The model under review builds one solid part; all positions refer to its coordinate system, in mm. Face numbers are marked on the shaded views. A direction names the side the tool comes from. Round coordinates to 2 decimals unless told otherwise and drop trailing zeros. Order: outer loops, then holes, each group sorted by start corner. A loop starts at its lowest first (then second) coordinate and runs counter-clockwise, first axis right, second up.
1) To check wall thickness, follow L1, parallel to Y at x = -13.8, z = 6.25; L2, parallel to Y at x = 9, z = -1.25; L3, parallel to Z at x = 6, y = 9.5. State the ranges of each line that lie inside material, in increasing order.
2) Consider section D-D (x = -8). Give the boundary of the cut face in (y, z).
3) Consider section A-A (x = -13.8). Give the boundary of the cut face in (y, z).
4) Consider section C-C (z = 3.75). Give the boundary of the cut face in (x, y).
5) Clearance check with flat-ended pins moving along their axes: P1, Ø5, axis at y = 12.5, z = 5.5, coming from the -X side; P2, Ø1, axis at y = 11.5, z = 6.5, coming from the +X side; P3, Ø1.8, axis at x = 13.8, y = 25.4, coming from the +Z side; P4, Ø3, axis at x = -10, z = 12, coming from the +Y side. State where each tip first meets the part, or that it passes through.
6) Consider section B-B (y = 25.4). Give the boundary of the cut face in (x, z), then the cut area to 3 significant figures.
7) Mouldability with a two-part tool opening along X and no side actions: class the marked faces 4, 5, 6 and 7 as pulls with the +X half, pulls with the -X half, needs draft (parallel to the pull), parting line crosses it, or undercut.
8) Machinability: for the marked faces 1, 2 and 3, which of the approach directions +Z, -Z, +X, -X, +Y, -Y give a long, thin tool a straight path to every point of the face, cutting with its end or side? Answer none if there is none.
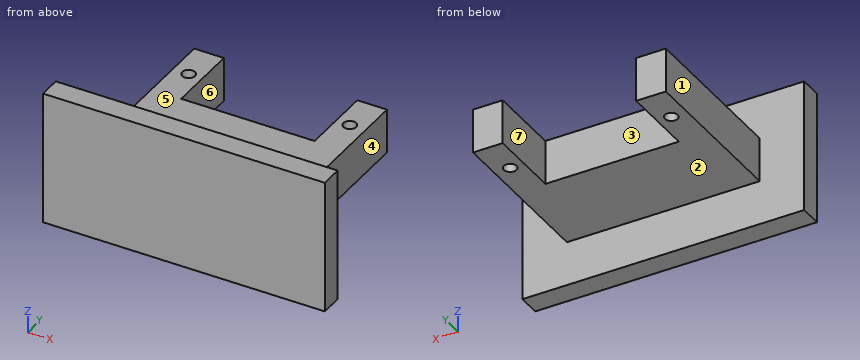
from build123d import *

# Parameters (mm, degrees)
BOSS_EXTRUDE4_DEPTH  = 7.62
SKETCH7_W            = 48.26
SKETCH7_H            = 22.86
BOSS_EXTRUDE5_DEPTH  = 3.81
M2_CLEARANCE_HOLE1_D = 2.2


with BuildPart() as part:
    # Sketch6 → Boss-Extrude4 (new body)
    with BuildSketch(Plane.XY):
        Polygon((-11.43, 19.05), (11.43, 19.05), (11.43, 31.75), (16.51, 31.75), (16.51, 0), (-16.51, 0), (-16.51, 31.75), (-11.43, 31.75), align=None)
    extrude(amount=BOSS_EXTRUDE4_DEPTH)

    # Sketch7 → Boss-Extrude5 (add)
    with BuildSketch(Plane(origin=(0, 0, 0), x_dir=(1, 0, 0), z_dir=(0, 1, 0))):
        with Locations((0, -3.81)):
            Rectangle(SKETCH7_W, SKETCH7_H)
    extrude(amount=BOSS_EXTRUDE5_DEPTH)

    # M2 Clearance Hole1 (through all)
    with Locations(Plane(origin=(0, 0, 0), x_dir=(-1, 0, 0), z_dir=(0, 0, -1))):
        with Locations((-13.8, 25.4), (13.8, 25.4)):
            Hole(M2_CLEARANCE_HOLE1_D / 2)


solid = part.part
Answer below:
1. L1: y = 0 to 24.3, 26.5 to 31.75
1. L2: y = 0 to 3.81
1. L3: z = 0 to 7.62
2. outline: (0, -7.62) - (3.81, -7.62) - (3.81, 0) - (19.05, 0) - (19.05, 7.62) - (3.81, 7.62) - (3.81, 15.24) - (0, 15.24) - close
3. outline: (0, -7.62) - (3.81, -7.62) - (3.81, 0) - (24.3, 0) - (24.3, 7.62) - (3.81, 7.62) - (3.81, 15.24) - (0, 15.24) - close; (26.5, 0) - (31.75, 0) - (31.75, 7.62) - (26.5, 7.62) - close
4. outline: (-24.13, 0) - (24.13, 0) - (24.13, 3.81) - (16.51, 3.81) - (16.51, 31.75) - (11.43, 31.75) - (11.43, 19.05) - (-11.43, 19.05) - (-11.43, 31.75) - (-16.51, 31.75) - (-16.51, 3.81) - (-24.13, 3.81) - close; hole circle Ø2.2 at (-13.8, 25.4); hole circle Ø2.2 at (13.8, 25.4)
5. P1: stops at x = -16.51
5. P2: stops at x = 16.51
5. P3: passes through
5. P4: stops at y = 3.81
6. outline: (-16.51, 0) - (-14.9, 0) - (-14.9, 7.62) - (-16.51, 7.62) - close; (-12.7, 0) - (-11.43, 0) - (-11.43, 7.62) - (-12.7, 7.62) - close; (11.43, 0) - (12.7, 0) - (12.7, 7.62) - (11.43, 7.62) - close; (14.9, 0) - (16.51, 0) - (16.51, 7.62) - (14.9, 7.62) - close
6. area: 43.9 mm2
7. face 4: pulls with the +X half
7. face 5: needs draft
7. face 6: undercut
7. face 7: undercut
8. face 1: +Z, -Z, -X, +Y
8. face 2: -Z, +X, -X, +Y
8. face 3: +Z, -Z, +Y
